Work out the finished part from the listing and answer in its coordinate system (mm). Face numbers are marked on the shaded views. A direction names the side the tool comes from. Coordinates: 2 decimals unless noted, no trailing zeros. Write each loop counter-clockwise with the first axis right and the second up, starting at its lowest first coordinate (ties: lowest second). Pieces come first, ordered by that corner, then holes. Notation, with made-up numbers: (-21.75, 87.5) - (29.25, 87.5) arc R19 ccw to (29.25, 91.5) - close; hole circle Ø9 at (42.5, 65). An arc over 180 degrees is marked (long way). Use CSV: the item, a comma, the result in double quotes. Start each with the question number.
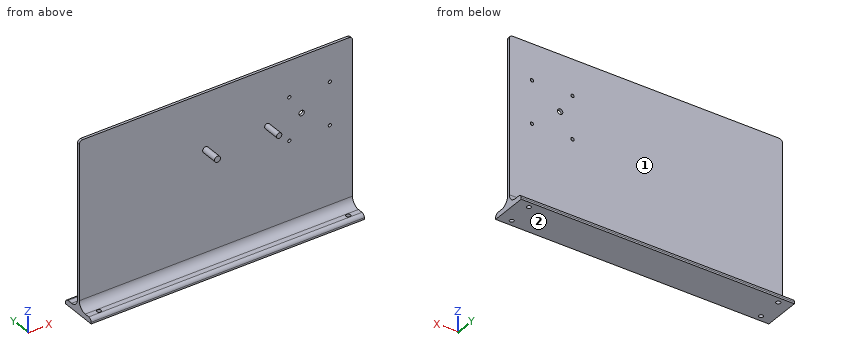
from build123d import *

# Parameters (mm, degrees)
F0_W      = 406.4
F0_H      = 254
F1_DEPTH  = 3.81
F2_W      = 406.4
F2_H      = 54.61
F3_DEPTH  = 7.62
F4_R      = 12.7
F5_R      = 5.08
F6_R      = 2.413
F6_R_2    = 3.96748
F7_DEPTH  = 29.211
F8_R      = 3.9624
F9_DEPTH  = 25.4
F10_R     = 4.445
F11_DEPTH = 25.4
F13_D     = 6.35


with BuildPart() as f1:
    # F0 (on Front) → F1 (new body)
    with BuildSketch(Plane.XZ):
        with Locations((203.2, 127)):
            Rectangle(F0_W, F0_H)
    extrude(amount=F1_DEPTH)

    # F2 (on face) → F3 (join)
    with BuildSketch(Plane(origin=(0, 0, 0), x_dir=(1, 0, 0), z_dir=(0, 0, -1))):
        with Locations((203.2, 1.905)):
            Rectangle(F2_W, F2_H)
    extrude(amount=-F3_DEPTH)

    # F4
    f4_edges = [f1.edges().sort_by_distance(p)[0] for p in [
        (203.2, 0, 7.62),
        (203.2, -3.81, 7.62),
    ]]
    fillet(f4_edges, radius=F4_R)

    # F5
    f5_edges = [f1.edges().sort_by_distance(p)[0] for p in [
        (203.2, -29.21, 7.62),
        (203.2, 25.4, 7.62),
        (406.4, -1.905, 254),
        (0, -1.905, 254),
    ]]
    fillet(f5_edges, radius=F5_R)

    # F6 (on face) → F7 (cut, through all)
    with BuildSketch(Plane.XZ.offset(3.81)):
        with Locations((312.4034767258, 200.2879581752)):
            Circle(F6_R)
        with Locations((372.7284767258, 200.2879581752)):
            Circle(F6_R)
        with Locations((312.4034767258, 136.7879581752)):
            Circle(F6_R)
        with Locations((372.7284767258, 136.7879581752)):
            Circle(F6_R)
        with Locations((330.7422767258, 170.3159581752)):
            Circle(F6_R_2)
    extrude(amount=-F7_DEPTH, mode=Mode.SUBTRACT)

    # F8 (on face) → F9 (join)
    with BuildSketch(Plane.XZ.offset(3.81)):
        with Locations((279.654, 170.3159581752)):
            Circle(F8_R)
    extrude(amount=F9_DEPTH)

    # F10 (on face) → F11 (join)
    with BuildSketch(Plane.XZ.offset(3.81)):
        with Locations((187.96, 170.3159581752)):
            Circle(F10_R)
    extrude(amount=F11_DEPTH)

    # F13 (through all)
    with Locations(Plane.XY.offset(7.62)):
        with Locations((388.62, 16.51), (388.62, -20.32), (17.78, 16.51), (17.78, -20.32)):
            Hole(F13_D / 2)


solid = f1.part
Item 1: Each of these flat-tipped pins is pushed along its axis until it touches: pin 1 (8 mm diameter, centred on x = 91, z = 203, fed in from +Y); pin 2 (8.5 mm diameter, centred on x = 17.78, y = 16.51, fed in from +Z); pin 3 (7.5 mm diameter, centred on x = 372.73, z = 200.29, fed in from -Y). Where does it stop, or does it pass through?
Item 2: Which of the six approach directions +Z, -Z, +X, -X, +Y, -Y give full straight-line access (tool end or side, diameter ignored) to the marked faces 1 and 2?
Item 3: A cutting plane is placed at B-B (z = 104). Determine the outline of the cut face in (x, y), then the cut area to 3 significant figures.
Item 4: Straight lines are drawn through the part: probe 1 along X at (y, z) = (-20, 5); probe 2 along Z at (x, y) = (38, 12); probe 3 along Y at (x, z) = (17.78, 4) (3 decimals). For each, find the intervals that lie inside material, in ascending order. Write a range as [from, to].
Item 5: A cutting plane is placed at A-A (x = 187.96). Determine the outline of the cut face in (y, z), then the cut area to 3 significant figures.
Item 6: A cutting plane is placed at C-C (y = -11). Determine the outline of the cut face in (x, z) (3 decimals), then the cut area to 3 significant figures.
Item 7: A cutting plane is placed at D-D (x = 253). Determine the outline of the cut face in (y, z).
Calculated:
1,pin 1,"stops at y = 0"
1,pin 2,"stops at z = 7.63"
1,pin 3,"stops at y = -3.81"
2,face 1,"+Z, +X, -X, +Y"
2,face 2,"-Z, +X, -X, +Y, -Y"
3,outline,"(0, -3.81) - (406.4, -3.81) - (406.4, 0) - (0, 0) - close"
3,area,"1,550 mm²"
4,probe 1,"x = [0, 14.62], [20.94, 385.46], [391.78, 406.4]"
4,probe 2,"z = [0, 7.64]"
4,probe 3,"y = [-28.996, -23.495], [-17.145, 13.335], [19.685, 25.186]"
5,outline,"(-29.21, 0) - (25.4, 0) - (25.4, 2.54) arc R5.08 ccw to (20.32, 7.62) - (12.7, 7.62) arc R12.7 cw to (0, 20.32) - (0, 254) - (-3.81, 254) - (-3.81, 174.76) - (-29.21, 174.76) - (-29.21, 165.87) - (-3.81, 165.87) - (-3.81, 20.32) arc R12.7 cw to (-16.51, 7.62) - (-24.13, 7.62) arc R5.08 ccw to (-29.21, 2.54) - close"
5,area,"1,640 mm²"
6,outline,"(0, 0) - (406.4, 0) - (406.4, 8.878) - (0, 8.878) - close; circle Ø8.89 at (187.96, 170.316); circle Ø7.925 at (279.654, 170.316)"
6,area,"3,720 mm²"
7,outline,"(-29.21, 0) - (25.4, 0) - (25.4, 2.54) arc R5.08 ccw to (20.32, 7.62) - (12.7, 7.62) arc R12.7 cw to (0, 20.32) - (0, 254) - (-3.81, 254) - (-3.81, 20.32) arc R12.7 cw to (-16.51, 7.62) - (-24.13, 7.62) arc R5.08 ccw to (-29.21, 2.54) - close"
